Work out the finished part from the listing and answer in its coordinate system (mm). A direction names the side the tool comes from. Give positions to 0.01 mm unless a question says otherwise; leave off trailing zeros. Order: outer loops, then holes, each group sorted by start corner. A loop starts at its lowest first (then second) coordinate and runs counter-clockwise, first axis right, second up. Notation, with made-up numbers: (-12.5, 21.25) - (21.5, 21.25) arc R34 ccw to (21.5, 51.25) - close; hole circle Ø9 at (18.5, 58). An arc over 180 degrees is marked (long way). Put each result on its own line as item: value.
```python
from build123d import *

# Parameters (mm, degrees)
F0_R     = 9.7055451223
F0_R_2   = 9.741664506
F0_R_3   = 9.6722617748
F0_R_4   = 8.6511366969
F0_R_5   = 9.6722557952
F1_DEPTH = 3.048


with BuildPart() as f1:
    # F0 (on Front) → F1 (new body)
    with BuildSketch(Plane.XZ):
        with BuildLine():
            ThreePointArc((3.8066026136, 38.808027463), (-26.1927234435, 28.8876177218), (-38.9942716181, 0))
            ThreePointArc((-38.9942716181, 0), (-26.1927225437, -28.8876185377), (3.8066050311, -38.8080272259))
            ThreePointArc((3.8066050311, -38.8080272259), (28.8876185377, -26.1927225437), (38.9942716181, 0))
            ThreePointArc((38.9942716181, 0), (28.8876177218, 26.1927234435), (3.8066026136, 38.808027463))
        make_face()
        Circle(F0_R, mode=Mode.SUBTRACT)
        with BuildLine():
            Line((-54.198741575, 127.3070507144), (-38.9942716181, 0))
            ThreePointArc((-38.9942716181, 0), (-26.1927234435, 28.8876177218), (3.8066026136, 38.808027463))
            Line((3.8066026136, 38.808027463), (43.6851335777, 34.8964187714))
            Line((43.6851335777, 34.8964187714), (58.0401596038, 141.6868133715))
            ThreePointArc((58.0401596038, 141.6868133715), (7.4420102551, 91.4013122397), (-54.198741575, 127.3070507144))
        make_face()
        with BuildLine():
            ThreePointArc((38.9942716181, 0), (28.8876185377, -26.1927225437), (3.8066050311, -38.8080272259))
            Line((3.8066050311, -38.8080272259), (135.7471495867, -25.8662320197))
            ThreePointArc((135.7471495867, -25.8662320197), (109.880917567, 0), (135.7471495867, 25.8662320197))
            Line((135.7471495867, 25.8662320197), (43.6851335777, 34.8964187714))
            Line((43.6851335777, 34.8964187714), (38.9942716181, 0))
        make_face()
        with BuildLine():
            Line((43.6851335777, 34.8964187714), (3.8066026136, 38.808027463))
            ThreePointArc((3.8066026136, 38.808027463), (28.8876177218, 26.1927234435), (38.9942716181, 0))
            Line((38.9942716181, 0), (43.6851335777, 34.8964187714))
        make_face()
        with BuildLine():
            Line((-57.8981825428, 158.2824757208), (-54.198741575, 127.3070507144))
            ThreePointArc((-54.198741575, 127.3070507144), (7.4420102551, 91.4013122397), (58.0401596038, 141.6868133715))
            ThreePointArc((58.0401596038, 141.6868133715), (58.4315346455, 145.5790412778), (58.5621873175, 149.4887142024))
            ThreePointArc((58.5621873175, 149.4887142024), (4.409397464, 207.8846643822), (-57.8981825428, 158.2824757208))
        make_face()
        with Locations((0, 149.4887142024)):
            Circle(F0_R_2, mode=Mode.SUBTRACT)
        with BuildLine():
            ThreePointArc((-57.8981825428, 158.2824757208), (-58.1489409856, 142.5438999028), (-54.198741575, 127.3070507144))
            Line((-54.198741575, 127.3070507144), (-57.8981825428, 158.2824757208))
        make_face()
        with BuildLine():
            ThreePointArc((135.7471495867, 25.8662320197), (109.880917567, 0), (135.7471495867, -25.8662320197))
            ThreePointArc((135.7471495867, -25.8662320197), (154.0373376515, -18.2901880649), (161.6133816064, 0))
            ThreePointArc((161.6133816064, 0), (154.0373376515, 18.2901880649), (135.7471495867, 25.8662320197))
        make_face()
        with Locations((135.7471495867, 0)):
            Circle(F0_R_3, mode=Mode.SUBTRACT)
        with BuildLine():
            Line((-36.0279004475, 347.1542968414), (-57.8981825428, 158.2824757208))
            ThreePointArc((-57.8981825428, 158.2824757208), (4.409397464, 207.8846643822), (58.5621873175, 149.4887142024))
            ThreePointArc((58.5621873175, 149.4887142024), (58.4315346455, 145.5790412778), (58.0401596038, 141.6868133715))
            Line((58.0401596038, 141.6868133715), (60.2709891258, 158.2824757208))
            Line((60.2709891258, 158.2824757208), (35.9735681678, 347.599410979))
            ThreePointArc((35.9735681678, 347.599410979), (36.1947916427, 345.2956505186), (36.2686330263, 342.9824709892))
            ThreePointArc((36.2686330263, 342.9824709892), (-2.0893828703, 306.7740711238), (-36.0279004475, 347.1542968414))
        make_face()
        with Locations((-24.9003618956, 294.7882115841)):
            Circle(F0_R_4, mode=Mode.SUBTRACT)
        with BuildLine():
            ThreePointArc((35.9735681678, 347.599410979), (-0.2242089383, 379.2504109906), (-36.0279004475, 347.1542968414))
            ThreePointArc((-36.0279004475, 347.1542968414), (-2.0893828703, 306.7740711238), (36.2686330263, 342.9824709892))
            ThreePointArc((36.2686330263, 342.9824709892), (36.1947916427, 345.2956505186), (35.9735681678, 347.599410979))
        make_face()
        with Locations((0, 342.9824709892)):
            Circle(F0_R_5, mode=Mode.SUBTRACT)
    extrude(amount=F1_DEPTH)


solid = f1.part
```
(1) Section A-A, the plane x = 0 is taken. Write down the section's boundary in (y, z), then the cut area to 3 significant figures.
Geometry check:
outline: (-3.05, -38.99) - (0, -38.99) - (0, -9.71) - (-3.05, -9.71) - close; (-3.05, 9.71) - (0, 9.71) - (0, 139.75) - (-3.05, 139.75) - close; (-3.05, 159.23) - (0, 159.23) - (0, 333.31) - (-3.05, 333.31) - close; (-3.05, 352.65) - (0, 352.65) - (0, 379.25) - (-3.05, 379.25) - close
area: 1,100 mm²
(2) Given pin 1 (1.5 mm diameter, centred on x = 92, y = -2.5, fed in from +Z); pin 2 (1 mm diameter, centred on x = 76, y = -2, fed in from +Z); pin 3 (15.5 mm diameter, centred on x = 0, z = 149.49, fed in from +Y), each flat-ended and moving along its own axis, determine where each tip first touches the part or whether it passes through.
Geometry check:
pin 1: stops at z = 30.23
pin 2: stops at z = 31.78
pin 3: passes through
(3) Straight lines are drawn through the part: line 1 (Z direction, x = 0, y = -1); line 2 (X direction, y = -0.75, z = -1); line 3 (X direction, y = -2.05, z = 0.5). For each, find the intervals that lie inside material, in ascending order.
Geometry check:
line 1: z = -38.99 to -9.71, 9.71 to 139.75, 159.23 to 333.31, 352.65 to 379.25
line 2: x = -38.98 to -9.65, 9.65 to 126.13, 145.37 to 161.59
line 3: x = -39.05 to -9.69, 9.69 to 126.09, 145.41 to 161.61
(4) Section C-C, the plane y = -1.15 is taken. Write down the section's boundary in (x, z).
Geometry check:
outline: (-57.9, 158.28) arc R58.56 ccw to (-54.2, 127.31) - (-38.99, 0) arc R38.99 ccw to (3.81, -38.81) - (135.75, -25.87) arc R25.87 ccw to (135.75, 25.87) - (43.69, 34.9) - (60.27, 158.28) - (35.97, 347.6) arc R36.27 ccw to (-36.03, 347.15) - close; hole circle Ø17.3 at (-24.9, 294.79); hole circle Ø19.48 at (0, 149.49); hole circle Ø19.41 at (0, 0); hole circle Ø19.34 at (0, 342.98); hole circle Ø19.34 at (135.75, 0)
(5) Section B-B, the plane x = 48 is taken. Write down the section's boundary in (y, z).
Geometry check:
outline: (-3.05, -34.47) - (0, -34.47) - (0, 34.47) - (-3.05, 34.47) - close; (-3.05, 67) - (0, 67) - (0, 253.89) - (-3.05, 253.89) - close
(6) Determine the mould class of faces 1 (the face through (5.2, -1.5, 351.14)), 2 (the face through (-20.908, -1.503, 287.113)), 3 (the face through (68.85, -1.5, -32.43)), 4 (the face through (0.512, -1.503, 379.247)) for opening direction X: pulls with the +X half, pulls with the -X half, needs draft (parallel to the pull), parting line crosses it, or undercut.
Geometry check:
face 1: undercut
face 2: undercut
face 3: pulls with the +X half
face 4: parting line crosses it
(7) Section D-D, the plane z = 178.5 is taken. Write down the section's boundary in (x, y).
Geometry check:
outline: (-55.56, -3.05) - (57.68, -3.05) - (57.68, 0) - (-55.56, 0) - close
(8) A tool of negligible diameter and unlimited length cuts with its end or side. For faces 5 (the face through (90.36, -1.5, 30.32)), 6 (the face through (-46.81, -1.5, 254.04)), from which of +Z, -Z, +X, -X, +Y, -Y can it reach the whole face along a straight path? Write none if from no direction.
Geometry check:
face 5: +X, +Y, -Y
face 6: +Z, -X, +Y, -Y
